Solid Edge part; units mm, degrees
sketch "Sketch1" plane through (0, 0, 0) normal (0, 0, 1) x (1, 0, 0)
  line L0 (-18, -27.5) -> (18, -27.5)
  line L1 (18, -27.5) -> (18, -21.7)
  arc A0 (18, -21.7) -> (19.7, -20) centre (19.7, -21.7) cw
  line L2 (19.7, -20) -> (33.3, -20)
  arc A1 (33.3, -20) -> (35, -18.3) centre (33.3, -18.3) ccw
  line L3 (35, -18.3) -> (35, 18.3)
  arc A2 (33.3, 20) -> (35, 18.3) centre (33.3, 18.3) cw
  line L4 (33.3, 20) -> (19.7, 20)
  arc A3 (18, 21.7) -> (19.7, 20) centre (19.7, 21.7) ccw
  line L5 (18, 21.7) -> (18, 27.5)
  line L6 (18, 27.5) -> (-18, 27.5)
  line L7 (-18, 27.5) -> (-18, 21.7)
  arc A4 (-19.7, 20) -> (-18, 21.7) centre (-19.7, 21.7) ccw
  line L8 (-19.7, 20) -> (-33.3, 20)
  arc A5 (-35, 18.3) -> (-33.3, 20) centre (-33.3, 18.3) cw
  line L9 (-35, 18.3) -> (-35, -18.3)
  arc A6 (-35, -18.3) -> (-33.3, -20) centre (-33.3, -18.3) ccw
  line L10 (-33.3, -20) -> (-19.7, -20)
  arc A7 (-19.7, -20) -> (-18, -21.7) centre (-19.7, -21.7) cw
  line L11 (-18, -21.7) -> (-18, -27.5)
extrude "Protrusion1" add sketch "Sketch1" along normal blind 8
sketch "Sketch2" plane through (0, -27.5, 4) normal (0, -1, 0) x (1, 0, 0)
  line L0 (-11.1, 0.8) -> (-17.9, 0.8)
  line L1 (-17.9, 0.8) -> (-17.9, -4)
  line L2 (-17.9, -4) -> (-11.1, -4)
  line L3 (-11.1, -4) -> (-11.1, 0.8)
  line L4 (11.1, 0.8) -> (17.9, 0.8)
  line L5 (17.9, 0.8) -> (17.9, -4)
  line L6 (17.9, -4) -> (11.1, -4)
  line L7 (11.1, -4) -> (11.1, 0.8)
extrude "ExtrudedProtrusion_2" add sketch "Sketch2" along normal blind 3.5
sketch "Sketch3" plane through (0, 27.5, 4) normal (0, 1, 0) x (-1, 0, 0)
  line L0 (-17.9, 0.8) -> (-11.1, 0.8)
  line L1 (-11.1, 0.8) -> (-11.1, -4)
  line L2 (-11.1, -4) -> (-17.9, -4)
  line L3 (-17.9, -4) -> (-17.9, 0.8)
extrude "ExtrudedProtrusion_3" add sketch "Sketch3" along normal blind 3.5
sketch "Sketch4" plane through (0, 0, 0) normal (0, 0, -1) x (0, 1, 0)
  arc A0 (-27.5, -8) -> (-27.5, -11) centre (-27.5, -9.5) cw
  line L0 (-27.5, -8) -> (-27.5, -11)
  arc A1 (-27.5, 11) -> (-27.5, 8) centre (-27.5, 9.5) cw
  line L1 (-27.5, 8) -> (-27.5, 11)
  arc A2 (27.5, -11) -> (27.5, -8) centre (27.5, -9.5) cw
  line L2 (27.5, -8) -> (27.5, -11)
  arc A3 (27.5, 8) -> (27.5, 11) centre (27.5, 9.5) cw
  line L3 (27.5, 8) -> (27.5, 11)
extrude "ExtrudedCutout_2" cut sketch "Sketch4" against normal blind 8
sketch "Sketch5" plane through (0, 27.5, 4) normal (0, 1, 0) x (-1, 0, 0)
  line L0 (11.1, 0.8) -> (17.9, 0.8)
  line L1 (17.9, 0.8) -> (17.9, -4)
  line L2 (17.9, -4) -> (11.1, -4)
  line L3 (11.1, -4) -> (11.1, 0.8)
extrude "ExtrudedProtrusion_4" add sketch "Sketch5" along normal blind 3.5
sketch "Sketch6" plane through (0, 0, 8) normal (0, 0, 1) x (-1, 0, 0)
  arc A0 (-1.5998, 20.0476) -> (1.5998, 20.0476) centre (0, 20.0254) ccw
  arc A1 (2.725, 21.5) -> (1.5998, 20.0476) centre (1.225, 21.5) cw
  line L0 (2.725, 23) -> (2.725, 21.5)
  arc A2 (1.5998, 24.4524) -> (2.725, 23) centre (1.225, 23) cw
  line L1 (1.5998, 27.5) -> (1.5998, 24.4524)
  line L2 (0, 27.5) -> (1.5998, 27.5)
  line L3 (0, 27.5) -> (-1.6, 27.5)
  line L4 (-1.6, 27.5) -> (-1.6, 24.4524)
  arc A3 (-1.6, 24.4524) -> (-2.725, 23) centre (-1.225, 23) ccw
  line L5 (-2.725, 23) -> (-2.725, 21.5)
  arc A4 (-2.725, 21.5) -> (-1.5998, 20.0476) centre (-1.225, 21.5) ccw
  arc A5 (-1.5998, -20.0476) -> (1.5998, -20.0476) centre (0, -20.0254) cw
  arc A6 (2.725, -21.5) -> (1.5998, -20.0476) centre (1.225, -21.5) ccw
  line L6 (2.725, -23) -> (2.725, -21.5)
  arc A7 (1.5998, -24.4524) -> (2.725, -23) centre (1.225, -23) ccw
  line L7 (1.5998, -27.5) -> (1.5998, -24.4524)
  line L8 (0, -27.5) -> (1.5998, -27.5)
  line L9 (0, -27.5) -> (-1.6, -27.5)
  line L10 (-1.6, -27.5) -> (-1.6, -24.4524)
  arc A8 (-1.6, -24.4524) -> (-2.725, -23) centre (-1.225, -23) cw
  line L11 (-2.725, -23) -> (-2.725, -21.5)
  arc A9 (-2.725, -21.5) -> (-1.5998, -20.0476) centre (-1.225, -21.5) cw
extrude "Cutout1" cut sketch "Sketch6" against normal up to next
sketch "Sketch7" plane through (0, 0, 0) normal (0, 0, -1) x (0, -1, 0)
  circle A0 centre (16, 27) radius 1.25
  circle A1 centre (-16, 27) radius 1.25
  circle A2 centre (-16, -27) radius 1.25
  circle A3 centre (16, -27) radius 1.25
extrude "Cutout2" cut sketch "Sketch7" against normal through all
properties material "Polycarbonate"
Source: CAD feature listing. Evaluate the final solid. Frame: model axes, mm. A direction names the side the tool comes from. Give positions to 0.01 mm unless a question says otherwise; leave off trailing zeros. Write each loop counter-clockwise with the first axis right and the second up, starting at its lowest first coordinate (ties: lowest second). Pieces come first, ordered by that corner, then holes.
1. Access query for faces 4 (the face through (18, 25, 4)), 5 (the face through (-11.1, -29, 2)), 6 (the face through (2.725, 22, 4)), 7 (the face through (-18, 25, 4)). Directions: +Z, -Z, +X, -X, +Y, -Y. A direction counts if a zero-diameter tool reaches every point of the face in a straight line with its end or side. Return the directions, or none.
2. Section query C-C (x = -12). Return the cut outline in (y, z).
3. Pull-direction query (Y, two-part tool) for faces 1 (the face through (2.419, 23.908, 4.056)), 2 (the face through (15, -31, 2)), 3 (the face through (-14, -29, 4.8)); classes: +Y half, -Y half, draft (parallel to the pull), parting line (faces both ways), or undercut.
4. Section query B-B (x = -27). Return the cut outline in (y, z), then the cut area to 3 significant figures.
5. Material intervals for line 1 along X through (y, z) = (16, 3.25); line 2 along Y through (x, z) = (-27, 5.75); line 3 along X through (y, z) = (23, 5.75) (3 decimals), sorted ascending.
6. Section query D-D (x = 0). Return the cut outline in (y, z).
7. First-contact query: pin 1 (0.9 mm diameter, centred on y = 25.5, z = 4.5, fed in from -X); pin 2 (4 mm diameter, centred on x = 18.5, z = 4.5, fed in from +Y); pin 3 (1.2 mm diameter, centred on y = 22.5, z = 3, fed in from +X); pin 4 (1.8 mm diameter, centred on y = -29, z = 2, fed in from +X). Flat tips, straight axial feed; report the tip coordinate or a pass-through.
8. Section query A-A (y = 16). Return the cut outline in (x, z), then the cut area to 3 significant figures.
Output values:
1. face 4: +Z, -Z, +X, +Y
1. face 5: +Z, -Z, -Y
1. face 6: +Z, -Z
1. face 7: +Z, -Z, -X, +Y
2. outline: (-31, 0) - (31, 0) - (31, 4.8) - (27.5, 4.8) - (27.5, 8) - (-27.5, 8) - (-27.5, 4.8) - (-31, 4.8) - close
3. face 1: undercut
3. face 2: -Y half
3. face 3: draft
4. outline: (-20, 0) - (-17.25, 0) - (-17.25, 8) - (-20, 8) - close; (-14.75, 0) - (14.75, 0) - (14.75, 8) - (-14.75, 8) - close; (17.25, 0) - (20, 0) - (20, 8) - (17.25, 8) - close
4. area: 280 mm2
5. line 1: x = -35 to -28.25, -25.75 to 25.75, 28.25 to 35
5. line 2: y = -20 to -17.25, -14.75 to 14.75, 17.25 to 20
5. line 3: x = -18 to -2.725, 2.725 to 18
6. outline: (-18.43, 0) - (18.43, 0) - (18.43, 8) - (-18.43, 8) - close
7. pin 1: stops at x = -18
7. pin 2: stops at y = 31
7. pin 3: stops at x = 18
7. pin 4: stops at x = 17.9
8. outline: (-35, 0) - (-28.25, 0) - (-28.25, 8) - (-35, 8) - close; (-25.75, 0) - (25.75, 0) - (25.75, 8) - (-25.75, 8) - close; (28.25, 0) - (35, 0) - (35, 8) - (28.25, 8) - close
8. area: 520 mm2
